Autodesk Inventor part; units mm, degrees
ref_plane "YZ Plane" through (0, 0, 0) normal (1, 0, 0) x (0, 1, 0)
ref_plane "XZ Plane" through (0, 0, 0) normal (0, 1, 0) x (-1, 0, 0)
ref_plane "XY Plane" through (0, 0, 0) normal (0, 0, 1) x (1, 0, 0)
sketch "Sketch1" plane through (0, 0, 0) normal (1, 0, 0) x (0, 1, 0)
  line L0 (0, 0) -> (0, 60)
  line L1 (0, 60) -> (11.2, 60)
  line L2 (11.2, 60) -> (11.2, 0)
  line L3 (11.2, 0) -> (0, 0)
  dimension "d2" = 60
  dimension "d4" = 11.2
extrude "Extrusion1" add sketch "Sketch1" along normal blind 25
sketch "Sketch2" plane through (0, 11.2, 60) normal (0, 1, 0) x (1, 0, 0)
  circle A0 centre (6, 53) radius 3
  point P0 (0, 60)
  dimension "d7" = 6
  dimension "d8" = 6
  dimension "d9" = 7
extrude "Extrusion2" cut sketch "Sketch2" against normal blind 20
pattern_linear "Rectangular Pattern1" count 2 spacing 46 along (0, 0, 1) count 2 spacing 13 along (1, 0, 0) of "Extrusion2"
properties part number "BK10_3030_Mount"
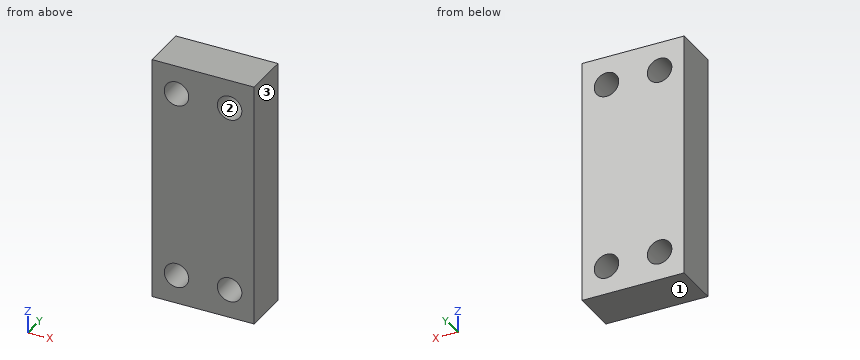
Work out the finished part from the listing and answer in its coordinate system (mm). Face numbers are marked on the shaded views. Round coordinates to 2 decimals unless told otherwise and drop trailing zeros. Write each loop counter-clockwise with the first axis right and the second up, starting at its lowest first coordinate (ties: lowest second). Pieces come first, ordered by that corner, then holes. Notation, with made-up numbers: (38, 14.5) -> (63, 14.5) arc R35 cw to (63, 48.5) -> close; hole circle Ø9 at (88.25, 89.25). An arc over 180 degrees is marked (long way). Write each question's results on one line, items separated by ' | '.
Item 1: Find the intervals of material crossed by line 1 along Z through (x, y) = (19, 6); line 2 along X through (y, z) = (8.75, 53); line 3 along Z through (x, y) = (17.5, 2), in increasing order. Write a range as [from, to].
Result set:
line 1: [0, 4], [10, 50], [56, 60] | line 2: [0, 3], [9, 16], [22, 25] | line 3: [0, 4.4], [9.6, 50.4], [55.6, 60]
Item 2: A cutting plane is placed at B-B, the plane y = 7.75. Determine the outline of the cut face in (x, z).
Result set:
outline: (0, 0) -> (25, 0) -> (25, 60) -> (0, 60) -> close; hole circle Ø6 at (6, 7); hole circle Ø6 at (6, 53); hole circle Ø6 at (19, 7); hole circle Ø6 at (19, 53)
Item 3: A cutting plane is placed at C-C, the plane z = 53. Determine the outline of the cut face in (x, y), plus the area to 3 significant figures.
Result set:
outline: (0, 0) -> (3, 0) -> (3, 11.2) -> (0, 11.2) -> close; (9, 0) -> (16, 0) -> (16, 11.2) -> (9, 11.2) -> close; (22, 0) -> (25, 0) -> (25, 11.2) -> (22, 11.2) -> close | area: 146 mm^2
Item 4: The mould has two halves that part along X. Classify the marked faces 1, 2 and 3: +X half, -X half, draft (parallel to the pull), parting line (faces both ways), or undercut.
Result set:
face 1: draft | face 2: undercut | face 3: +X half
Item 5: A cutting plane is placed at A-A, the plane x = 6. Determine the outline of the cut face in (y, z).
Result set:
outline: (0, 0) -> (11.2, 0) -> (11.2, 4) -> (0, 4) -> close; (0, 10) -> (11.2, 10) -> (11.2, 50) -> (0, 50) -> close; (0, 56) -> (11.2, 56) -> (11.2, 60) -> (0, 60) -> close
Item 6: Flat-ended cylindrical pins translate along their axes: P1, Ø6, axis at x = 2.5, y = 2.5, coming from the -Z side; P2, Ø3.5, axis at x = 6, z = 7, coming from the -Y side. Find the tip coordinate at first contact, or state that the pin passes through.
Result set:
P1: z = 0 | P2: through
